Verification items for the finished model (mm, model axes). A direction names the side the tool comes from. Give positions to 0.01 mm unless a question says otherwise; leave off trailing zeros. Write each loop counter-clockwise with the first axis right and the second up, starting at its lowest first coordinate (ties: lowest second). Pieces come first, ordered by that corner, then holes. Notation, with made-up numbers: (87.25, 63.5) - (114.25, 63.5) arc R16 cw to (114.25, 94.5) - close; hole circle Ø10 at (58.25, 62). An arc over 180 degrees is marked (long way). Answer as a JSON object with one key per item and string values. Group by question number.
Item 1: Scan lines: line 1 along Z through (x, y) = (2.75, 5); line 2 along Y through (x, z) = (-3.25, 5); line 3 along Z through (x, y) = (-2.25, 21). Record each from-to range of solid material in increasing order. Write a range as [from, to].
Item 2: Tool access check on faces 5 (the face through (0.672, -18.108, 4.93)), 6 (the face through (-9.4, -9, 5)), 7 (the face through (1.6, -13, 5)), 8 (the face through (2, 26.6, 5)), 9 (the face through (-2, 10, 2.25)). Record the directions out of +Z, -Z, +X, -X, +Y, -Y that give a thin tool (end or side, any length) a straight path to the whole face; none if there is none.
Item 3: Draft check along Z on faces 1 (the face through (-8, -7.774, 5)), 2 (the face through (0, 29, 9)), 3 (the face through (0, 29, 1)), 4 (the face through (2, 10, 3.4)). Enter one of: +Z half, -Z half, draft (parallel to the pull), parting line (faces both ways), or undercut.
Item 4: Sectioned sample at A-A, the plane y = 1.5. Record the boundary of the cut face in (x, z), and give its area (3 significant figures).
Item 5: Go/stop test with flat-tipped pins: pin 1 (4 mm diameter, centred on x = -1, z = 4, fed in from -Y); pin 2 (4.5 mm diameter, centred on y = 9.5, z = 3.5, fed in from -X); pin 3 (1.1 mm diameter, centred on x = -10, z = 4, fed in from +Y). Record where each tip stops, or that it passes through.
Item 6: Sectioned sample at B-B, the plane z = 9.5. Record the boundary of the cut face in (x, y).
```python
from build123d import *

# Parameters (mm, degrees)
PAD_DEPTH       = 10
POCKET_DEPTH    = 5
CHAMFER_SIZE    = 1
POCKET001_DEPTH = 4.4
CHAMFER001_SIZE = 2


with BuildPart() as part:
    # Sketch → Pad (new body)
    with BuildSketch(Plane.XY):
        with BuildLine():
            Line((0, 30), (4, 30))
            Line((4, 30), (4, 0))
            Line((4, 0), (4, -19))
            Line((4, -19), (-2.75, -17.191343))
            Line((-2.75, -17.191343), (-2.063716, -16.002664))
            ThreePointArc((1.6, -13.5), (-0.51688, -14.334081), (-2.063716, -16.002664))
            Line((1.6, -13.5), (1.6, -11.542586))
            ThreePointArc((1.6, -11.542586), (-0.147655, -12.333269), (-1.656853, -13.517244))
            Line((-11.107107, -22.967498), (-1.656853, -13.517244))
            Line((-11.814214, -22.260391), (-11.107107, -22.967498))
            Line((-10.4, -20.846177), (-11.814214, -22.260391))
            Line((-10.4, -10), (-10.4, -20.846177))
            Line((-9.4, -10), (-10.4, -10))
            Line((-9.4, -8.774099), (-9.4, -10))
            Line((-8.4, -7.774099), (-9.4, -8.774099))
            Line((-7.4, -7.774099), (-8.4, -7.774099))
            Line((-2.363961, -12.810138), (-7.4, -7.774099))
            ThreePointArc((1.6, -10.5), (-0.53166, -11.398235), (-2.363961, -12.810138))
            Line((1.6, -10.5), (1.6, -10))
            Line((1.6, -10), (-4.4, -10))
            Line((-4.4, 0), (-4.4, -10))
            Line((-4.4, 0), (-4.4, 30))
            Line((-4.4, 30), (0, 30))
        make_face()
    extrude(amount=PAD_DEPTH)

    # Sketch001 → Pocket (cut)
    with BuildSketch(Plane.YZ):
        with BuildLine():
            ThreePointArc((-5, 6.6), (-6.6, 5), (-5, 3.4))
            Line((-5, 3.4), (25, 3.4))
            ThreePointArc((25, 3.4), (26.6, 5), (25, 6.6))
            Line((-5, 6.6), (25, 6.6))
        make_face()
    extrude(amount=POCKET_DEPTH, mode=Mode.SUBTRACT)

    # Chamfer
    chamfer_edges = [part.edges().sort_by_distance(p)[0] for p in [
        (-4.4, -10, 5),
    ]]
    chamfer(chamfer_edges, length=CHAMFER_SIZE)

    # Sketch002 (on DatumPlane) → Pocket001 (cut)
    with BuildSketch(Plane(origin=(-4.4, 0, 0), x_dir=(0, -1, 0), z_dir=(-1, 0, 0))):
        Polygon((6.587713, 7.75), (8.175426, 5), (6.587713, 2.25), (-26.587713, 2.25), (-28.175426, 5), (-26.587713, 7.75), align=None)
    extrude(amount=-POCKET001_DEPTH, mode=Mode.SUBTRACT)

    # Chamfer001
    chamfer001_edges = [part.edges().sort_by_distance(p)[0] for p in [
        (-2.2, 30, 10),
        (-2.2, 30, 0),
    ]]
    chamfer(chamfer001_edges, length=CHAMFER001_SIZE)


solid = part.part
```
Geometry check:
{
 "1": {"line 1": "[0, 3.4], [6.6, 10]", "line 2": "[-15.11, -11.92], [-10, -8.18], [28.18, 30]", "line 3": "[0, 2.25], [7.75, 10]"},
 "2": {"face 5": "+Z, -Z, -Y", "face 6": "+Z, -Z, -X, +Y", "face 7": "+Z, -Z", "face 8": "+X, -X", "face 9": "-X"},
 "3": {"face 1": "draft", "face 2": "+Z half", "face 3": "-Z half", "face 4": "undercut"},
 "4": {"outline": "(-4.4, 0) - (4, 0) - (4, 3.4) - (0, 3.4) - (0, 2.25) - (-4.4, 2.25) - close; (-4.4, 7.75) - (0, 7.75) - (0, 6.6) - (4, 6.6) - (4, 10) - (-4.4, 10) - close", "area": "47.0 mm^2"},
 "5": {"pin 1": "y = -18.2", "pin 2": "x = -4.4", "pin 3": "y = -10"},
 "6": {"outline": "(-11.81, -22.26) - (-11.11, -22.97) - (-1.66, -13.52) arc R8 cw to (1.6, -11.54) - (1.6, -13.5) arc R5.12 ccw to (-2.06, -16) - (-2.75, -17.19) - (4, -19) - (4, 28.5) - (-4.4, 28.5) - (-4.4, -9) - (-3.4, -10) - (1.6, -10) - (1.6, -10.5) arc R9 ccw to (-2.36, -12.81) - (-7.4, -7.77) - (-8.4, -7.77) - (-9.4, -8.77) - (-9.4, -10) - (-10.4, -10) - (-10.4, -20.85) - close"}
}
